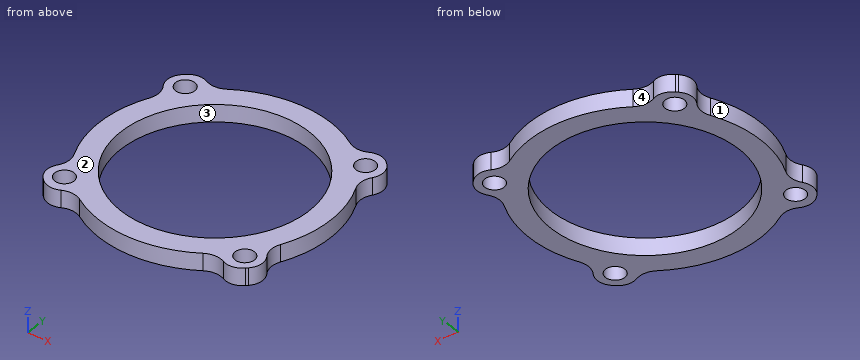
Autodesk Inventor part; units mm, degrees
ref_plane "YZ Plane" through (0, 0, 0) normal (1, 0, 0) x (0, 1, 0)
ref_plane "XZ Plane" through (0, 0, 0) normal (0, 1, 0) x (-1, 0, 0)
ref_plane "XY Plane" through (0, 0, 0) normal (0, 0, 1) x (1, 0, 0)
sketch "Sketch6" plane through (0, 0, 0) normal (0, 0, 1) x (1, 0, 0)
  circle A0 centre (3.9228, -14.5408) radius 10.15
  line L0 (10.903848, -34.81) -> (-10.903848, -34.81)
  line L1 (54.2, 8.803848) -> (54.2, -8.803848)
  circle A1 centre (3.9228, -14.5408) radius 16.4625
  circle A2 centre (19.9228, -0.5408) radius 1.5
  circle A3 centre (3.9228, -14.5408) radius 18.415
  line L2 (3.9228, -14.5408) -> (3.9228, -8.803848)
  line L3 (3.9228, -14.5408) -> (9.053444, -14.5408)
  circle A4 centre (3.9228, -14.5408) radius 20.2692
  line L4 (17.090037, 0.869078) -> (19.9228, 3.701841)
  line L5 (21.032601, -3.67364) -> (24.165441, -0.5408)
  line L6 (19.9228, 3.701841) -> (24.165441, -0.5408)
  line L7 (3.9228, -14.5408) -> (19.9228, -0.5408) construction
  line L8 (-12.0772, 3.701841) -> (-16.319841, -0.5408)
  line L9 (-13.187001, -3.67364) -> (-16.319841, -0.5408)
  circle A5 centre (-12.0772, -0.5408) radius 1.5
  line L10 (-9.244437, 0.869078) -> (-12.0772, 3.701841)
  line L11 (-9.244437, -29.950678) -> (-12.0772, -32.783441)
  line L12 (-12.0772, -32.783441) -> (-16.319841, -28.5408)
  circle A6 centre (-12.0772, -28.5408) radius 1.5
  line L13 (-13.187001, -25.40796) -> (-16.319841, -28.5408)
  line L14 (17.090037, -29.950678) -> (19.9228, -32.783441)
  line L15 (19.9228, -32.783441) -> (24.165441, -28.5408)
  line L16 (21.032601, -25.40796) -> (24.165441, -28.5408)
  circle A7 centre (19.9228, -28.5408) radius 1.5
  line L17 (24.165441, -28.5408) -> (18.258589, -22.633949)
  line L18 (19.9228, -32.783441) -> (14.388092, -27.248733)
  line L19 (-12.0772, -32.783441) -> (-6.542492, -27.248733)
  line L20 (-16.319841, -28.5408) -> (-10.412989, -22.633949)
  line L21 (-16.319841, -0.5408) -> (-10.412989, -6.447651)
  line L22 (-12.0772, 3.701841) -> (-6.542492, -1.832867)
  point P0 (0, 0)
  point P1 (0, 0)
  dimension "d53" = 32.925
  dimension "d54" = 3
  dimension "d55" = 36.83
  dimension "d56" = 14
  dimension "d57" = 16
  dimension "d58" = 45
  dimension "d59" = 3
  dimension "d60" = 3
  dimension "d61" = 3
extrude "Extrusion4" add sketch "Sketch6" along normal blind 3 contours A1 L22 A3 L17 | A1 L21 A3 L22 | L17 A3 L18 A1 | A1 L20 A3 L21 | L22 A4 A2 L17 A3 | A3 L21 A4 A5 L22 | L18 A3 L19 A1 | L17 A4 A7 L18 A3 | A1 L19 A3 L20 | A3 L20 A4 L21 | A4 A5 L9 L8 L10 | L18 A4 L19 A3 | L16 L15 L14 A4 A7 | A3 L19 A4 A6 L20 | L4 L6 L5 A4 A2 | A5 A4 | A4 A5 | A7 A4 | A4 A7 | A4 A6 L11 L12 L13 | A4 A2 | A2 A4 | A6 A4 | A4 A6
fillet "Fillet4" radius 3.5 8 edges at (-9.2444, 0.8691, 1.5) (-13.187, -3.6736, 1.5) (-13.187, -25.408, 1.5) (-9.2444, -29.9507, 1.5) (17.09, 0.8691, 1.5) (21.0326, -3.6736, 1.5) (21.0326, -25.408, 1.5) (17.09, -29.9507, 1.5)
fillet "Fillet5" radius 3 8 edges at (19.9228, 3.7018, 1.5) (24.1654, -0.5408, 1.5) (24.1654, -28.5408, 1.5) (19.9228, -32.7834, 1.5) (-16.3198, -28.5408, 1.5) (-12.0772, -32.7834, 1.5) (-16.3198, -0.5408, 1.5) (-12.0772, 3.7018, 1.5)
sketch "Sketch7" plane through (0, 0, 3) normal (0, 0, 1) x (1, 0, 0)
  circle A0 centre (3.9228, -14.5408) radius 10.15
  line L0 (10.903848, -34.81) -> (-10.903848, -34.81)
  line L1 (54.2, 8.803848) -> (54.2, -8.803848)
  circle A1 centre (3.9228, -14.5408) radius 16.4625
  circle A2 centre (19.9228, -0.5408) radius 1.5
  circle A3 centre (3.9228, -14.5408) radius 18.415
  line L2 (3.9228, -14.5408) -> (3.9228, -8.803848)
  line L3 (3.9228, -14.5408) -> (9.053444, -14.5408)
  circle A4 centre (3.9228, -14.5408) radius 20.2692
  line L4 (17.090037, 0.869078) -> (19.9228, 3.701841)
  line L5 (21.032601, -3.67364) -> (24.165441, -0.5408)
  line L6 (19.9228, 3.701841) -> (24.165441, -0.5408)
  line L7 (3.9228, -14.5408) -> (19.9228, -0.5408) construction
  line L8 (-12.0772, 3.701841) -> (-16.319841, -0.5408)
  line L9 (-13.187001, -3.67364) -> (-16.319841, -0.5408)
  circle A5 centre (-12.0772, -0.5408) radius 1.5
  line L10 (-9.244437, 0.869078) -> (-12.0772, 3.701841)
  line L11 (-9.244437, -29.950678) -> (-12.0772, -32.783441)
  line L12 (-12.0772, -32.783441) -> (-16.319841, -28.5408)
  circle A6 centre (-12.0772, -28.5408) radius 1.5
  line L13 (-13.187001, -25.40796) -> (-16.319841, -28.5408)
  line L14 (17.090037, -29.950678) -> (19.9228, -32.783441)
  line L15 (19.9228, -32.783441) -> (24.165441, -28.5408)
  line L16 (21.032601, -25.40796) -> (24.165441, -28.5408)
  circle A7 centre (19.9228, -28.5408) radius 1.5
  line L17 (24.165441, -28.5408) -> (18.258589, -22.633949)
  line L18 (19.9228, -32.783441) -> (14.388092, -27.248733)
  line L19 (-12.0772, -32.783441) -> (-6.542492, -27.248733)
  line L20 (-16.319841, -28.5408) -> (-10.412989, -22.633949)
  line L21 (-16.319841, -0.5408) -> (-10.412989, -6.447651)
  line L22 (-12.0772, 3.701841) -> (-6.542492, -1.832867)
  point P0 (0, 0)
  point P1 (0, 0)
  dimension "d66" = 32.925
  dimension "d67" = 3
  dimension "d68" = 36.83
  dimension "d69" = 14
  dimension "d70" = 16
  dimension "d71" = 45
  dimension "d72" = 3
  dimension "d73" = 3
  dimension "d74" = 3
hole "Hole3" at (-12.0772, -0.5408, 3) at (-12.0772, -28.5408, 3) at (19.9228, -28.5408, 3) at (19.9228, -0.5408, 3) direction (0, 0, -1) diameter 3.4036 depth 25.4 tip angle 118
properties part number "Cam.case.glassmount" material "Aluminum-6061"
Model file for the job. Use its own axes, mm. Face numbers are marked on the shaded views. Give positions to 0.01 mm unless a question says otherwise; leave off trailing zeros. Order: outer loops, then holes, each group sorted by start corner. A loop starts at its lowest first (then second) coordinate and runs counter-clockwise, first axis right, second up.
1) Mould opens along Y. For the marked faces 1, 2, 3 and 4 say: +Y half, -Y half, draft (parallel to the pull), parting line (faces both ways), or undercut.
2) Pin check, flat tips, straight feed: pin 1 (2.5 mm diameter, centred on x = -12.08, y = -28.54, fed in from +Z); pin 2 (6 mm diameter, centred on x = 0, y = -27.5, fed in from -Z); pin 3 (1.5 mm diameter, centred on x = 10.5, z = 0.5, fed in from +Y). Stop position of each tip, or through.
3) Wall check: probe 1 along Y at (x, z) = (3.5, 1.8); probe 2 along X at (y, z) = (0.5, 2.55); probe 3 along X at (y, z) = (-4, 0.6). Give the ranges that are in metal, low to high.
4) Saw through at D-D, the plane z = 2.3. Count the separate pieces of the cut face and the enclosed holes in it, then the cut area to 3 significant figures.
5) Saw through at A-A, the plane x = 11. Write the cut outline in (y, z).
6) Saw through at C-C, the plane y = -21.5. Write the cut outline in (x, z).
7) Saw through at B-B, the plane y = -27.5. Write the cut outline in (x, z).
Computed:
1. face 1: undercut
1. face 2: draft
1. face 3: undercut
1. face 4: +Y half
2. pin 1: passes through
2. pin 2: stops at z = 0
2. pin 3: stops at y = 4.87
3. probe 1: y = -34.81 to -31, 1.92 to 5.72
3. probe 2: x = -14.94 to -13.42, -10.73 to -2.77, 10.62 to 18.58, 21.27 to 22.78
3. probe 3: x = -14.03 to -8.72, 16.57 to 21.88
4. separate pieces: 1
4. enclosed holes: 5
4. area: 501 mm2
5. outline: (-33.53, 0) - (-29.4, 0) - (-29.4, 3) - (-33.53, 3) - close; (0.32, 0) - (4.45, 0) - (4.45, 3) - (0.32, 3) - close
6. outline: (-15.11, 0) - (-11, 0) - (-11, 3) - (-15.11, 3) - close; (18.84, 0) - (22.96, 0) - (22.96, 3) - (18.84, 3) - close
7. outline: (-15, 0) - (-13.42, 0) - (-13.42, 3) - (-15, 3) - close; (-10.73, 0) - (-6.23, 0) - (-6.23, 3) - (-10.73, 3) - close; (14.08, 0) - (18.58, 0) - (18.58, 3) - (14.08, 3) - close; (21.27, 0) - (22.84, 0) - (22.84, 3) - (21.27, 3) - close
